For this review, take the finished solid that the model builds, in its own axes (mm). Face numbers are marked on the shaded views. A direction names the side the tool comes from. Round coordinates to 2 decimals unless told otherwise and drop trailing zeros. Order: outer loops, then holes, each group sorted by start corner. A loop starts at its lowest first (then second) coordinate and runs counter-clockwise, first axis right, second up. Notation, with made-up numbers: (-16.75, -3.75) - (12.25, -3.75) arc R22 ccw to (12.25, 15.25) - close; hole circle Ø11 at (61.5, 84.25). An arc over 180 degrees is marked (long way). One line per question, with ' | ' between items.
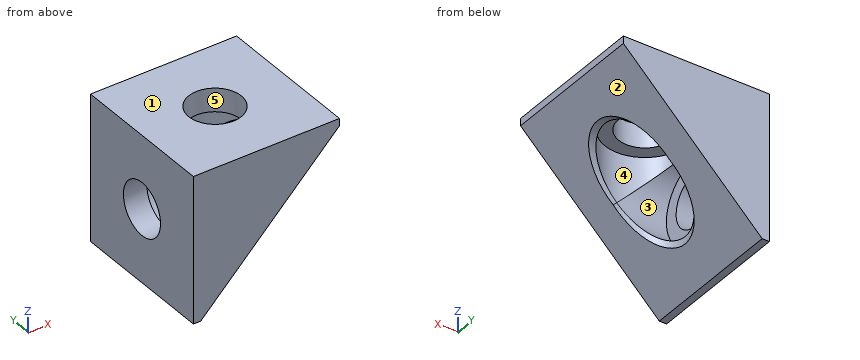
```python
from build123d import *

# Parameters (mm, degrees)
BOSS_EXTRUDE1_DEPTH     = 10
CUT_EXTRUDE1_REACH      = 32
SKETCH3_R               = 3.6
CUT_EXTRUDE3_REACH      = 35.2
CUT_EXTRUDE3_START      = -3.2
SKETCH3_4_R             = 5.5
SKETCH3_4_R_2           = 3.6
CUT_EXTRUDE2_REACH      = 32
CUT_EXTRUDE2_END_RADIUS = 5.5
SKETCH4_R               = 3.6
CUT_EXTRUDE4_REACH      = 35.2
CUT_EXTRUDE4_START      = -3.2
SKETCH4_3_R             = 5.5
SKETCH4_3_R_2           = 3.6


with BuildPart() as part:
    # Sketch2 → Boss-Extrude1 (new, symmetric)
    with BuildSketch(Plane(origin=(0, 0, 0), x_dir=(1, 0, 0), z_dir=(0, 1, 0))):
        Polygon((0, 0), (0, 20), (1, 20), (20, 1), (20, 0), align=None)
    extrude(amount=BOSS_EXTRUDE1_DEPTH, both=True)

    # Cut-Extrude1: up to this plane
    cut_extrude1_end = Plane(origin=(1, 10, -20), z_dir=(-0.7071067811865476, 0, 0.7071067811865476))
    # Sketch3 → Cut-Extrude1 (cut, up to the surface)
    with BuildSketch(Plane.XY, mode=Mode.PRIVATE) as cut_extrude1_sk1:
        with Locations((10, 0)):
            Circle(SKETCH3_R)
    cut_extrude1_tool1 = split(extrude(cut_extrude1_sk1.sketch, amount=-CUT_EXTRUDE1_REACH, mode=Mode.PRIVATE), bisect_by=cut_extrude1_end, keep=Keep.BOTH, mode=Mode.PRIVATE)
    add(cut_extrude1_tool1.solids().sort_by_distance((10, 0, 0))[0], mode=Mode.SUBTRACT)

    # Cut-Extrude3: up to this plane
    cut_extrude3_end = Plane(origin=(1, 10, -20), z_dir=(-0.7071067811865476, 0, 0.7071067811865476))
    # Sketch3_4 → Cut-Extrude3 (cut, up to the surface)
    with BuildSketch(Plane.XY.offset(CUT_EXTRUDE3_START), mode=Mode.PRIVATE) as cut_extrude3_sk1:
        with Locations((10, 0)):
            Circle(SKETCH3_4_R)
        with Locations((10, 0)):
            Circle(SKETCH3_4_R_2, mode=Mode.SUBTRACT)
    cut_extrude3_tool1 = split(extrude(cut_extrude3_sk1.sketch, amount=-CUT_EXTRUDE3_REACH, mode=Mode.PRIVATE), bisect_by=cut_extrude3_end, keep=Keep.BOTH, mode=Mode.PRIVATE)
    add(cut_extrude3_tool1.solids().sort_by_distance((4.655563, 0, -3.2))[0], mode=Mode.SUBTRACT)

    # Cut-Extrude2: up to this cylinder (the profile starts outside it)
    cut_extrude2_end = Plane(origin=(10, 0, -10), z_dir=(0, 0, 1)) * Cylinder(CUT_EXTRUDE2_END_RADIUS, 76, mode=Mode.PRIVATE)
    # Sketch4 → Cut-Extrude2 (cut, up to the surface)
    with BuildSketch(Plane.ZY, mode=Mode.PRIVATE) as cut_extrude2_sk1:
        with Locations((-10, 0)):
            Circle(SKETCH4_R)
    cut_extrude2_tool1 = extrude(cut_extrude2_sk1.sketch, amount=-CUT_EXTRUDE2_REACH, mode=Mode.PRIVATE) - cut_extrude2_end
    add(cut_extrude2_tool1.solids().sort_by_distance((0, 0, -10))[0], mode=Mode.SUBTRACT)

    # Cut-Extrude4: up to this plane
    cut_extrude4_end = Plane(origin=(1, 10, -20), z_dir=(-0.7071067811865476, 0, 0.7071067811865476))
    # Sketch4_3 → Cut-Extrude4 (cut, up to the surface)
    with BuildSketch(Plane.ZY.offset(CUT_EXTRUDE4_START), mode=Mode.PRIVATE) as cut_extrude4_sk1:
        with Locations((-10, 0)):
            Circle(SKETCH4_3_R)
        with Locations((-10, 0)):
            Circle(SKETCH4_3_R_2, mode=Mode.SUBTRACT)
    cut_extrude4_tool1 = split(extrude(cut_extrude4_sk1.sketch, amount=-CUT_EXTRUDE4_REACH, mode=Mode.PRIVATE), bisect_by=cut_extrude4_end, keep=Keep.BOTH, mode=Mode.PRIVATE)
    add(cut_extrude4_tool1.solids().sort_by_distance((3.2, 0, -15.344437))[0], mode=Mode.SUBTRACT)


solid = part.part
```
(1) For the marked faces 4 and 5, list the 3-axis set-ups (+Z, -Z, +X, -X, +Y, -Y) from which the entire face can be reached by the end or side of a thin tool; tool diameter is ignored.
Output values:
face 4: -Z | face 5: +Z, -Z
(2) We need section C-C on z = -2.5. State the section outline as (x, y) points, plus the area to 3 significant figures.
Output values:
outline: (0, -10) - (18.5, -10) - (18.5, 10) - (0, 10) - close; hole circle Ø7.2 at (10, 0) | area: 329 mm^2
(3) Mouldability with a two-part tool opening along Z and no side actions: class the marked faces 1, 2 and 3 as released by +Z, released by -Z, zero draft, split by the parting line, or undercut.
Output values:
face 1: released by +Z | face 2: released by -Z | face 3: undercut
(4) For probe 1 along Y at (x, z) = (1.1, -10); probe 2 along Z at (x, y) = (6.5, 1.5); probe 3 along X at (y, z) = (-0.5, -2), list the stretches that pass through material, from the lowest coordinate up. Write a range as [from, to].
Output values:
probe 1: [-10, -3.6], [3.6, 10] | probe 2: [-3.2, 0] | probe 3: [0, 6.43], [13.57, 19]
(5) We need section A-A on x = 9.5. State the section outline as (y, z) points, plus the area to 3 significant figures.
Output values:
outline: (-10, -11.5) - (-5.48, -11.5) - (-5.48, -10.5) arc R5.5 cw to (-5.48, -9.5) - (-5.48, -3.2) - (-3.57, -3.2) - (-3.57, 0) - (-10, 0) - close; (3.57, -3.2) - (5.48, -3.2) - (5.48, -9.5) arc R5.5 cw to (5.48, -10.5) - (5.48, -11.5) - (10, -11.5) - (10, 0) - (3.57, 0) - close | area: 116 mm^2
(6) Insertion check: pin 1 (9 mm diameter, centred on x = 9, y = -1.5, fed in from -Z); pin 2 (6.5 mm diameter, centred on x = 10, y = 0, fed in from +Z); pin 3 (12 mm diameter, centred on x = 13.5, y = -7.5, fed in from -Z); pin 4 (3.5 mm diameter, centred on y = -1, z = -12, fed in from +X). Each pin has a flat end and moves straight along its axis. Give the tip position at first contact, or say it passes through.
Output values:
pin 1: z = -16.5 | pin 2: through | pin 3: z = -13.5 | pin 4: x = 3.2
(7) We need section D-D on x = 1.75. State the section outline as (y, z) points, plus the area to 3 significant figures.
Output values:
outline: (-10, -19.25) - (10, -19.25) - (10, 0) - (-10, 0) - close; hole circle Ø7.2 at (0, -10) | area: 344 mm^2
(8) We need section B-B on y = 0. State the section outline as (x, z) points, plus the area to 3 significant figures.
Output values:
outline: (0, -20) - (1, -20) - (4.5, -16.5) - (4.5, -15.5) - (3.2, -15.5) - (3.2, -13.6) - (0, -13.6) - close; (0, -6.4) - (3.2, -6.4) - (3.2, -4.5) - (4.5, -4.5) - (4.5, -3.2) - (6.4, -3.2) - (6.4, 0) - (0, 0) - close; (13.6, -3.2) - (15.5, -3.2) - (15.5, -4.5) - (16.5, -4.5) - (20, -1) - (20, 0) - (13.6, 0) - close | area: 72.8 mm^2
